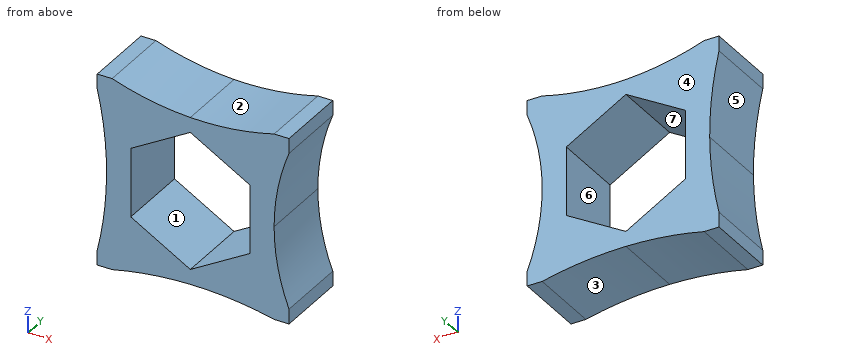
from build123d import *

# Parameters (mm, degrees)
F1_DEPTH = 10.033


with BuildPart() as f1:
    # F0 (on Front) → F1 (new body)
    with BuildSketch(Plane.XZ):
        with BuildLine():
            Line((11.43, 0), (8.128, 0))
            Line((8.128, 0), (8.128, -4.692703))
            Line((8.128, -4.692703), (0, -9.385406))
            Line((0, -9.385406), (-8.128, -4.692703))
            Line((-8.128, -4.692703), (-8.128, 0))
            Line((-8.128, 0), (-10.16, 0))
            Line((-10.16, 0), (-11.43, 0))
            ThreePointArc((-11.43, 0), (-11.769576, -5.36917), (-12.7, -10.668))
            Line((-12.7, -10.668), (-12.7, -12.7))
            Line((-12.7, -12.7), (-10.668, -12.7))
            ThreePointArc((-10.668, -12.7), (-5.36917, -11.769576), (0, -11.43))
            ThreePointArc((0, -11.43), (5.752665, -11.726018), (11.43, -12.7))
            Line((11.43, -12.7), (13.462, -12.7))
            Line((13.462, -12.7), (13.462, -11.684))
            Line((13.462, -11.684), (13.462, -10.668))
            ThreePointArc((13.462, -10.668), (11.942526, -5.4299), (11.43, 0))
        make_face()
        with BuildLine():
            Line((8.128, 4.692703), (8.128, 0))
            Line((8.128, 0), (11.43, 0))
            ThreePointArc((11.43, 0), (11.942526, 5.4299), (13.462, 10.668))
            Line((13.462, 10.668), (13.462, 11.684))
            Line((13.462, 11.684), (13.462, 12.7))
            Line((13.462, 12.7), (11.43, 12.7))
            ThreePointArc((11.43, 12.7), (5.763913, 11.624785), (0, 11.43))
            ThreePointArc((0, 11.43), (-5.407854, 12.058267), (-10.668, 13.462))
            Line((-10.668, 13.462), (-12.7, 13.462))
            Line((-12.7, 13.462), (-12.7, 11.43))
            ThreePointArc((-12.7, 11.43), (-11.726018, 5.752665), (-11.43, 0))
            Line((-11.43, 0), (-10.16, 0))
            Line((-10.16, 0), (-8.128, 0))
            Line((-8.128, 0), (-8.128, 4.692703))
            Line((-8.128, 4.692703), (0, 9.385406))
            Line((0, 9.385406), (8.128, 4.692703))
        make_face()
    extrude(amount=F1_DEPTH)


solid = f1.part
For this review, take the finished solid that the model builds, in its own axes (mm). Face numbers are marked on the shaded views. A direction names the side the tool comes from. Round coordinates to 2 decimals unless told otherwise and drop trailing zeros. Order: outer loops, then holes, each group sorted by start corner. A loop starts at its lowest first (then second) coordinate and runs counter-clockwise, first axis right, second up. Notation, with made-up numbers: M 39.25,-15.5 L 80.25,-15.5 A21 cw 80.25,4.5 Z; hole C 70.25,7 d7. An arc over 180 degrees is marked long. Use a Markdown table: item, result. Add a question column.
Item 1: Insertion check: pin 1 (3 mm diameter, centred on x = -8.5, y = -6, fed in from -Z); pin 2 (4.5 mm diameter, centred on y = -4.5, z = 2, fed in from -X); pin 3 (4 mm diameter, centred on y = -6, z = -0.5, fed in from -X). Each pin has a flat end and moves straight along its axis. Give the tip position at first contact, or say it passes through.
Item 2: To check wall thickness, follow line 1 along X through (y, z) = (-2.5, -6.5); line 2 along X through (y, z) = (-3.75, 3.5); line 3 along Z through (x, y) = (-2.75, -1.25). State the ranges of each line that lie inside material, in increasing order.
Item 3: Mouldability with a two-part tool opening along X and no side actions: class the marked faces 4, 5, 6 and 7 as released by +X, released by -X, zero draft, split by the parting line, or undercut.
Item 4: Tool access review of the marked faces 1, 2 and 3: name each direction out of +Z, -Z, +X, -X, +Y, -Y from which nothing blocks a thin tool from reaching the whole face with its end or side.
Item 5: Add section A-A, the plane y = -1.25. Give the boundary of the cut face in (x, z).
Item 6: Add section D-D, the plane x = -8.75. Give the boundary of the cut face in (y, z).
Item 7: Add section C-C, the plane x = -3. Give the boundary of the cut face in (y, z), then the cut area to 3 significant figures.
Item 8: Add section B-B, the plane z = -7.5. Give the boundary of the cut face in (x, y), then the cut area to 3 significant figures.
Geometry results:
| question | item | result |
|---|---|---|
| 1 | pin 1 | stops at z = -12.55 |
| 1 | pin 2 | stops at x = -11.58 |
| 1 | pin 3 | stops at x = -11.51 |
| 2 | line 1 | x = -11.92 to -5, 5 to 12.17 |
| 2 | line 2 | x = -11.53 to -8.13, 8.13 to 11.64 |
| 2 | line 3 | z = -11.53 to -7.8, 7.8 to 11.65 |
| 3 | face 4 | zero draft |
| 3 | face 5 | released by -X |
| 3 | face 6 | undercut |
| 3 | face 7 | undercut |
| 4 | face 1 | +Y, -Y |
| 4 | face 2 | +Z, +Y, -Y |
| 4 | face 3 | -Z, +Y, -Y |
| 5 | outline | M -12.7,-12.7 L -10.67,-12.7 A48.64 cw 0,-11.43 A48.64 cw 11.43,-12.7 L 13.46,-12.7 L 13.46,-10.67 A29.02 cw 13.46,10.67 L 13.46,12.7 L 11.43,12.7 A37.55 cw 0,11.43 A37.55 cw -10.67,13.46 L -12.7,13.46 L -12.7,11.43 A48.64 cw -11.43,0 A48.64 cw -12.7,-10.67 Z; hole M -8.13,-4.69 L 0,-9.39 L 8.13,-4.69 L 8.13,4.69 L 0,9.39 L -8.13,4.69 Z |
| 6 | outline | M -10.03,-12.29 L 0,-12.29 L 0,12.85 L -10.03,12.85 Z |
| 7 | outline | M -10.03,-11.55 L 0,-11.55 L 0,-7.65 L -10.03,-7.65 Z; M -10.03,7.65 L 0,7.65 L 0,11.68 L -10.03,11.68 Z |
| 7 | area | 79.5 mm² |
| 8 | outline | M -12.07,-10.03 L -3.27,-10.03 L -3.27,0 L -12.07,0 Z; M 3.27,-10.03 L 12.42,-10.03 L 12.42,0 L 3.27,0 Z |
| 8 | area | 180 mm² |
